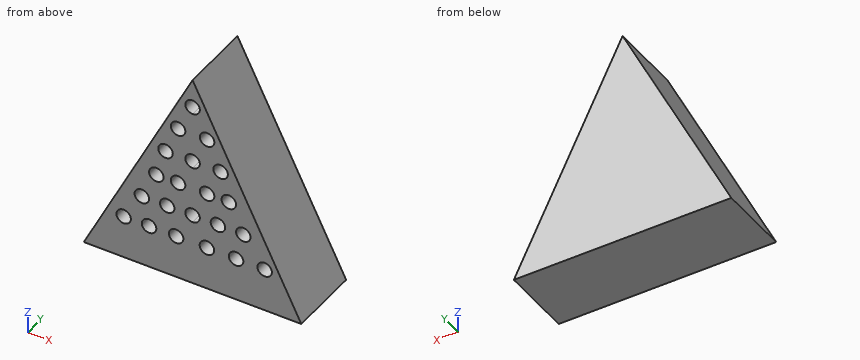
from build123d import *

# Parameters (mm, degrees)
F1_DEPTH = 25.4
F2_R     = 2.54
F3_DEPTH = 12.7


with BuildPart() as f1:
    # F0 (on Front) → F1 (new body)
    with BuildSketch(Plane.XZ):
        Polygon((5.74964, 36.402817), (-32.35036, -39.797183), (5.74964, -39.797183), (5.74964, 34.851611), align=None)
        Polygon((5.74964, 34.851611), (5.74964, -39.797183), (43.84964, -39.797183), (5.74964, 36.402817), align=None)
    extrude(amount=F1_DEPTH)

    # F2 (on face) → F3 (cut)
    with BuildSketch(Plane.XZ.offset(25.4)):
        with BuildLine():
            ThreePointArc((8.28964, 26.242817), (7.545691, 28.038868), (5.74964, 28.782817))
            Line((5.74964, 28.782817), (5.74964, 26.242817))
            Line((5.74964, 26.242817), (5.74964, 23.702817))
            ThreePointArc((5.74964, 23.702817), (7.545691, 24.446766), (8.28964, 26.242817))
        make_face()
        with BuildLine():
            ThreePointArc((8.28964, -14.397183), (7.545691, -12.601132), (5.74964, -11.857183))
            Line((5.74964, -11.857183), (5.74964, -14.397183))
            Line((5.74964, -14.397183), (5.74964, -16.937183))
            ThreePointArc((5.74964, -16.937183), (7.545691, -16.193234), (8.28964, -14.397183))
        make_face()
        with BuildLine():
            Line((5.74964, -14.397183), (5.74964, -11.857183))
            ThreePointArc((5.74964, -11.857183), (3.20964, -14.397183), (5.74964, -16.937183))
            Line((5.74964, -16.937183), (5.74964, -14.397183))
        make_face()
        with BuildLine():
            ThreePointArc((8.28964, 5.922817), (7.545691, 7.718868), (5.74964, 8.462817))
            Line((5.74964, 8.462817), (5.74964, 5.922817))
            Line((5.74964, 5.922817), (5.74964, 3.382817))
            ThreePointArc((5.74964, 3.382817), (7.545691, 4.126766), (8.28964, 5.922817))
        make_face()
        with BuildLine():
            Line((5.74964, 5.922817), (5.74964, 8.462817))
            ThreePointArc((5.74964, 8.462817), (3.20964, 5.922817), (5.74964, 3.382817))
            Line((5.74964, 3.382817), (5.74964, 5.922817))
        make_face()
        with BuildLine():
            Line((5.74964, 26.242817), (5.74964, 28.782817))
            ThreePointArc((5.74964, 28.782817), (3.20964, 26.242817), (5.74964, 23.702817))
            Line((5.74964, 23.702817), (5.74964, 26.242817))
        make_face()
        with Locations((0.66964, 16.082817)):
            Circle(F2_R)
        with Locations((10.82964, 16.082817)):
            Circle(F2_R)
        with Locations((-3.729841, 5.922817)):
            Circle(F2_R)
        with BuildLine():
            ThreePointArc((13.036175, 5.922817), (15.576175, 3.382817), (18.116175, 5.922817))
            ThreePointArc((18.116175, 5.922817), (15.576175, 8.462817), (13.036175, 5.922817))
        make_face()
        with Locations((0.66964, -4.237183)):
            Circle(F2_R)
        with Locations((-6.95036, -4.237183)):
            Circle(F2_R)
        with Locations((10.82964, -4.237183)):
            Circle(F2_R)
        with Locations((18.4496, -4.251403)):
            Circle(F2_R)
        with Locations((-3.140297, -14.379193)):
            Circle(F2_R)
        with Locations((-12.030297, -14.379193)):
            Circle(F2_R)
        with BuildLine():
            ThreePointArc((12.09964, -14.397183), (14.63964, -16.937183), (17.17964, -14.397183))
            ThreePointArc((17.17964, -14.397183), (14.63964, -11.857183), (12.09964, -14.397183))
        make_face()
        with BuildLine():
            ThreePointArc((20.988973, -14.455365), (23.528973, -16.995365), (26.068973, -14.455365))
            ThreePointArc((26.068973, -14.455365), (23.528973, -11.915365), (20.988973, -14.455365))
        make_face()
        with Locations((0, -24.557183)):
            Circle(F2_R)
        with Locations((-9.49036, -24.557183)):
            Circle(F2_R)
        with Locations((-18.397864, -24.557183)):
            Circle(F2_R)
        with Locations((10.773869, -24.557183)):
            Circle(F2_R)
        with Locations((20.98964, -24.557183)):
            Circle(F2_R)
        with Locations((31.00442, -24.557183)):
            Circle(F2_R)
    extrude(amount=-F3_DEPTH, mode=Mode.SUBTRACT)


solid = f1.part
Design review of the part built by this model. Coordinates are the model's own, in mm. Give positions to 0.01 mm unless a question says otherwise; leave off trailing zeros. Loops run counter-clockwise (first coordinate to the right, second up) from the corner with the lowest first, then second, coordinate; pieces in that order, holes last. Notation, with made-up numbers: (48.25, 51.5) - (75.25, 51.5) arc R30 ccw to (75.25, 75.5) - close; hole circle Ø5 at (76.25, -3.75). An arc over 180 degrees is marked (long way). Use CSV: the item, a comma, the result in double quotes. Start each with the question number.
1. Add section B-B (x = 10.5). State the section outline as (y, z) points, plus the area to 3 significant figures.
2. Add section D-D (z = -35). State the section outline as (x, y) points, plus the area to 3 significant figures.
3. Add section A-A (y = -19.5). Count the separate pieces of the cut face and the enclosed holes in it, plus the area to 3 significant figures.
4. Insertion check: P1, Ø1.5, axis at x = 11.5, z = -3, coming from the -Y side; P2, Ø12, axis at y = -17.5, z = -0.5, coming from the -X side; P3, Ø2, axis at y = -5.5, z = -18, coming from the -X side. Each pin has a flat end and moves straight along its axis. Give the tip position at first contact, or say it passes through.
5. Add section C-C (y = -4.5). State the section outline as (x, z) points, plus the area to 3 significant figures.
6. Wall thickness on L1, parallel to Z at x = 22, y = -24; L2, parallel to Z at x = 9, y = -14.25; L3, parallel to Z at x = -12.5, y = -16.25: over which ranges is each line inside the solid? List them lowest first.
Results found:
1,outline,"(-25.4, -39.8) - (0, -39.8) - (0, 26.9) - (-25.4, 26.9) - (-25.4, 18.6) - (-12.7, 18.6) - (-12.7, 13.56) - (-25.4, 13.56) - (-25.4, -1.72) - (-12.7, -1.72) - (-12.7, -6.76) - (-25.4, -6.76) - (-25.4, -22.03) - (-12.7, -22.03) - (-12.7, -27.08) - (-25.4, -27.08) - close"
1,area,"1,500 mm²"
2,outline,"(-29.95, -25.4) - (41.45, -25.4) - (41.45, 0) - (-29.95, 0) - close"
2,area,"1,810 mm²"
3,separate pieces,"1"
3,enclosed holes,"21"
3,area,"2,480 mm²"
4,P1,"stops at y = -12.7"
4,P2,"stops at x = -15.7"
4,P3,"stops at x = -21.95"
5,outline,"(-32.35, -39.8) - (43.85, -39.8) - (5.75, 36.4) - close"
5,area,"2,900 mm²"
6,L1,"z = -39.8 to -26.89, -22.23 to -16.48, -12.43 to 3.9"
6,L2,"z = -39.8 to -26.38, -22.74 to -6, -2.48 to 14.32, 17.84 to 29.9"
6,L3,"z = -39.8 to -16.88, -11.88 to -0.1"
